The model under review builds one solid part; all positions refer to its coordinate system, in mm. Face numbers are marked on the shaded views. Coordinates: 2 decimals unless noted, no trailing zeros. Loops run counter-clockwise (first coordinate to the right, second up) from the corner with the lowest first, then second, coordinate; pieces in that order, holes last. Notation, with made-up numbers: (12, 31.5) - (41, 31.5) arc R32 cw to (41, 65.5) - close; hole circle Ø8 at (10, -28.75). An arc over 180 degrees is marked (long way). One line per item, written item: value. Start each with the question number.
1. We need section C-C, the plane y = 24. Give the boundary of the cut face in (x, z).
2. Mouldability with a two-part tool opening along Z and no side actions: class the marked faces 1 and 2 as +Z half, -Z half, draft (parallel to the pull), parting line (faces both ways), or undercut.
3. Insertion check: P1, Ø1.5, axis at x = 47.5, y = 25.5, coming from the -Z side; P2, Ø6, axis at x = -44, z = -43, coming from the -Y side; P3, Ø10, axis at x = -22, y = 35, coming from the +Z side. Each pin has a flat end and moves straight along its axis. Give the tip position at first contact, or say it passes through.
4. To check wall thickness, follow line 1 (Z direction, x = 0, y = 57); line 2 (Z direction, x = 0, y = -12.35) (3 decimals). State the ranges of each line that lie inside material, in increasing order.
5. We need section B-B, the plane z = 11.5. Give the boundary of the cut face in (x, y), then the cut area to 3 significant figures.
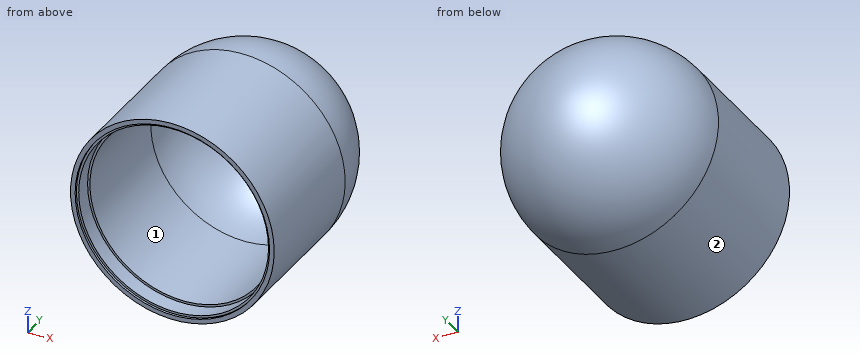
from build123d import *

# Parameters (mm, degrees)
SKETCH1_W           = 3.175
SKETCH1_H           = 12.7
SKETCH2_R           = 66.675
SKETCH2_R_2         = 65.0875
BOSS_EXTRUDE1_DEPTH = 11.1125


with BuildPart() as part:
    # Sketch1 → Revolve3 (revolve)
    with BuildSketch(Plane.XY):
        with BuildLine():
            Line((69.85, 0), (69.85, 76.2))
            ThreePointArc((69.85, 76.2), (49.391408666, 125.591408666), (0, 146.05))
            Line((0, 146.05), (0, 139.7))
            ThreePointArc((0, 139.7), (44.901280605, 121.101280605), (63.5, 76.2))
            Line((63.5, 76.2), (63.5, 0))
            Line((63.5, 0), (69.85, 0))
        make_face()
        with Locations((68.2625, -6.35)):
            Rectangle(SKETCH1_W, SKETCH1_H)
    revolve(axis=Axis((0, 146.05, 0), (0, -1, 0)))

    # Sketch2 → Boss-Extrude1 (add)
    with BuildSketch(Plane(origin=(0, 0, 0), x_dir=(-1, 0, 0), z_dir=(0, -1, 0))):
        Circle(SKETCH2_R)
        Circle(SKETCH2_R_2, mode=Mode.SUBTRACT)
    extrude(amount=BOSS_EXTRUDE1_DEPTH)


solid = part.part
Findings below:
1. outline: circle Ø139.7 at (0, 0); hole circle Ø127 at (0, 0)
2. face 1: undercut
2. face 2: parting line
3. P1: z = -51.9
3. P2: y = 0
3. P3: z = 67.75
4. line 1: -69.85 to -63.5, 63.5 to 69.85
4. line 2: -69.85 to -66.675, 66.675 to 69.85
5. outline: (-68.9, -12.7) - (-65.68, -12.7) - (-65.68, -11.11) - (-64.06, -11.11) - (-64.06, 0) - (-62.45, 0) - (-62.45, 76.2) arc R62.45 cw to (62.45, 76.2) - (62.45, 0) - (64.06, 0) - (64.06, -11.11) - (65.68, -11.11) - (65.68, -12.7) - (68.9, -12.7) - (68.9, 76.2) arc R68.9 ccw to (-68.9, 76.2) - close
5. area: 2,430 mm2
